Input: part model. Units: mm. Frame: model coordinates. A direction names the side the tool comes from. Round coordinates to 2 decimals unless told otherwise and drop trailing zeros. Write each loop counter-clockwise with the first axis right and the second up, starting at its lowest first coordinate (ties: lowest second). Pieces come first, ordered by that corner, then holes. Notation, with made-up numbers: (-30, -26) - (14, -26) arc R15 ccw to (14, -18) - close; hole circle Ø6 at (-9, -33.5). An arc over 180 degrees is marked (long way). Use one line per item in the form item = value.
Autodesk Inventor part; units mm, degrees
ref_plane "YZ Plane" through (0, 0, 0) normal (1, 0, 0) x (0, 1, 0)
ref_plane "XZ Plane" through (0, 0, 0) normal (0, 1, 0) x (-1, 0, 0)
ref_plane "XY Plane" through (0, 0, 0) normal (0, 0, 1) x (1, 0, 0)
sketch "Sketch1" plane through (0, 0, 0) normal (0, 0, 1) x (1, 0, 0)
  line L0 (40.3696, 0) -> (44.816, 0)
  line L1 (293.0054, 0) -> (287.9217, 0)
  arc A0 (0, 40.3696) -> (53.3921, 2.1581) centre (40.3696, 40.3696) ccw
  arc A1 (283.1915, 1.211) -> (333.375, 40.3696) centre (293.0054, 40.3696) ccw
  arc A2 (166.6875, 15.627) -> (44.816, 0) centre (166.3688, -464.9274) ccw
  arc A3 (287.9217, 0) -> (283.1915, 1.211) centre (166.3688, -464.9274) ccw
  arc A4 (53.3921, 2.1581) -> (44.816, 0) centre (166.3688, -464.9274) ccw
  arc A5 (287.9217, 0) -> (166.6875, 15.627) centre (166.3688, -464.9274) ccw
  line L2 (0, 40.3696) -> (0, 317.5)
  line L3 (333.375, 317.5) -> (333.375, 40.3696)
  line L4 (0, 317.5) -> (333.375, 317.5)
  line L5 (40.3696, 0) -> (293.0054, 0)
  point P0 (0, 0)
  point P1 (46.8129, 0.5175)
  dimension "d158" = 333.375
  dimension "d173" = 317.5
extrude "Extrusion1" add sketch "Sketch1" along normal blind 5.5563 contours A0 L2 L4 L3 A1 A5 A2
sketch "Sketch2" plane through (0, 0, 5.5563) normal (0, 0, 1) x (1, 0, 0)
  line L0 (43.8965, 34.0196) -> (47.5626, 40.3696)
  line L1 (43.8965, 46.7196) -> (47.5626, 40.3696)
  line L2 (36.5641, 46.7196) -> (43.8965, 46.7196)
  line L3 (36.5641, 34.0196) -> (43.8965, 34.0196)
  line L4 (36.5641, 46.7196) -> (32.898, 40.3696)
  line L5 (32.898, 40.3696) -> (36.5641, 34.0196)
  circle A0 centre (40.3696, 40.3696) radius 2.9337
  circle A1 centre (26.0449, 161.4785) radius 2.4066
  line L6 (0, 187.5234) -> (0, 40.3696)
  circle A2 centre (166.6875, 161.4785) radius 2.4066
  line L7 (333.375, 187.5234) -> (0, 187.5234)
  circle A3 centre (293.0054, 40.3696) radius 2.4066
  arc A4 (283.1915, 1.211) -> (333.375, 40.3696) centre (293.0054, 40.3696) ccw
  circle A5 centre (307.3301, 161.4785) radius 2.4066
  line L8 (333.375, 40.3696) -> (333.375, 187.5234)
  circle A6 centre (40.3696, 40.3696) radius 2.4066
  arc A7 (0, 40.3696) -> (46.8129, 0.5175) centre (40.3696, 40.3696) ccw
  line L9 (22.2394, 167.8285) -> (18.5732, 161.4785)
  line L10 (18.5732, 161.4785) -> (22.2394, 155.1285)
  line L11 (22.2394, 167.8285) -> (29.5718, 167.8285)
  line L12 (22.2394, 155.1285) -> (29.5718, 155.1285)
  line L13 (29.5718, 155.1285) -> (33.2379, 161.4785)
  line L14 (29.5718, 167.8285) -> (33.2379, 161.4785)
  circle A8 centre (26.0449, 161.4785) radius 2.9337
  point P0 (333.375, 40.3696)
  point P1 (283.1915, 1.211)
  point P2 (365.2681, 51.0131)
  point P3 (0, 0)
  point P4 (0, 0)
  dimension "d102" = 12.7
  dimension "d103" = 12.7
  dimension "d104" = 12.7
  dimension "d105" = 7.3323
  dimension "d106" = 7.3323
  dimension "d107" = 7.3323
  dimension "d108" = 7.3323
  dimension "d109" = 7.3323
  dimension "d110" = 7.3323
  dimension "d145" = 5.8674
  dimension "d160" = 333.375
  dimension "d161" = 12.7
  dimension "d162" = 12.7
  dimension "d163" = 12.7
  dimension "d164" = 7.3323
  dimension "d165" = 7.3323
  dimension "d166" = 7.3323
  dimension "d167" = 7.3323
  dimension "d168" = 7.3323
  dimension "d169" = 7.3323
  dimension "d170" = 5.8674
extrude "Extrusion2" cut sketch "Sketch2" against normal through all contours L3 L5 L4 L2 L1 L0 | A0 | A1 | A2 | A3 | A5 | A6 | L11 L14 L13 L12 L10 L9 | A8
sketch "Sketch6" plane through (0, 0, 5.5563) normal (0, 0, 1) x (1, 0, 0)
  ellipse E0 centre (224.6212, 89.9867) end of major axis (224.6174, 91.9867) minor radius 2
  ellipse E1 centre (224.6212, 57.9868) end of major axis (224.6139, 59.9867) minor radius 2
  line L0 (292.9982, 40.3696) -> (224.6212, 40.3696)
  line L1 (224.6212, 40.3696) -> (224.6212, 57.9868)
  ellipse E2 centre (108.7157, 89.9867) end of major axis (108.7119, 91.9867) minor radius 2
  ellipse E3 centre (108.7466, 57.9868) end of major axis (108.7392, 59.9867) minor radius 2
  line L2 (108.7466, 40.2597) -> (108.7466, 57.8769)
  circle A0 centre (224.6521, 73.9867) radius 4.699
  circle A1 centre (108.7466, 73.9867) radius 4.699
  line L3 (40.3696, 40.2597) -> (108.7466, 40.2597)
  circle A2 centre (293.0054, 40.3696) radius 2.4066
  point P0 (0, 0)
  dimension "d147" = 17.6171
  dimension "d150" = 17.6171
  dimension "d152" = 9.398
  dimension "d153" = 9.398
  dimension "d171" = 31.9999
  dimension "d172" = 31.9999
extrude "Extrusion7" cut sketch "Sketch6" against normal through all contours A0 | A1
properties part number "FTC Outside Panels" material "Wood (Oak)"
(1) Draft query along X for faces 1 (the face through (164, 196, 0)), 2 (the face through (105.432, 11.748, 2.739)). Return one class per face: released by +X, released by -X, zero draft, split by the parting line, or undercut.
Derived:
face_1 = zero draft
face_2 = undercut
(2) Cut plane A-A on z = 2.6. Output: boundary loops of the cut face in (x, y) (1 decimal), then the cut area to 3 significant figures.
Derived:
outline = (0, 40.4) arc R40.4 ccw to (46.8, 0.5) arc R480.6 cw to (166.7, 15.6) arc R480.6 cw to (283.2, 1.2) arc R40.4 ccw to (333.4, 40.4) - (333.4, 317.5) - (0, 317.5) - close; hole (18.6, 161.5) - (22.2, 155.1) - (29.6, 155.1) - (33.2, 161.5) - (29.6, 167.8) - (22.2, 167.8) - close; hole (32.9, 40.4) - (36.6, 34) - (43.9, 34) - (47.6, 40.4) - (43.9, 46.7) - (36.6, 46.7) - close; hole circle Ø9.4 at (108.7, 74); hole circle Ø4.8 at (166.7, 161.5); hole circle Ø9.4 at (224.7, 74); hole circle Ø4.8 at (293, 40.4); hole circle Ø4.8 at (307.3, 161.5)
area = 102,000 mm^2
(3) Cut plane B-B on x = 159. Output: boundary loops of the cut face in (y, z).
Derived:
outline = (15.57, 0) - (317.5, 0) - (317.5, 5.56) - (15.57, 5.56) - close
(4) Material intervals for L1, parallel to X at y = 73, z = 3.7 (3 decimals); L2, parallel to Y at x = 42, z = 2.9; L3, parallel to X at y = 41, z = 0.2 (3 decimals), sorted ascending.
Derived:
L1 = 0 to 104.152, 113.341 to 220.058, 229.246 to 333.375
L2 = 0.03 to 34.02, 46.72 to 317.5
L3 = 0 to 33.262, 47.199 to 290.683, 295.328 to 333.375
(5) Access query for faces 3 (the face through (113.09, 72.19, 2.82)), 4 (the face through (224.56, 12.09, 2.74)). Directions: +Z, -Z, +X, -X, +Y, -Y. A direction counts if a zero-diameter tool reaches every point of the face in a straight line with its end or side. Return the directions, or none.
Derived:
face_3 = +Z, -Z
face_4 = +Z, -Z, -Y
(6) First-contact query: pin 1 Ø15 at (x, y) = (108.75, 73.99) entering from +Z. Flat tip, straight axial feed; report the tip coordinate or a pass-through.
Derived:
pin_1 = 5.56
(7) Cut plane C-C on y = 23.5. Output: boundary loops of the cut face in (x, z), then the cut area to 3 significant figures.
Derived:
outline = (3.69, 0) - (329.68, 0) - (329.68, 5.56) - (3.69, 5.56) - close
area = 1,810 mm^2
